Read the model definition and answer for the solid it produces. Units are mm, in the model's axes. A direction names the side the tool comes from. Coordinates: 2 decimals unless noted, no trailing zeros. Write each loop counter-clockwise with the first axis right and the second up, starting at its lowest first coordinate (ties: lowest second). Pieces come first, ordered by that corner, then holes. Notation, with made-up numbers: (88.5, -9.75) - (133.5, -9.75) arc R13 ccw to (133.5, 7.25) - close; hole circle Ø5 at (54, -21.75). An arc over 180 degrees is marked (long way). Use a Markdown table: item, result.
from build123d import *

# Parameters (mm, degrees)
F1_DEPTH = 171.45
F2_R     = 5.5626
F3_DEPTH = 72.873041
F4_R     = 3.9751
F5_DEPTH = 76.972204
F6_R     = 6.35


with BuildPart() as f1:
    # F0 (on Top) → F1 (new body)
    with BuildSketch(Plane.XY):
        with BuildLine():
            Line((0, 0), (0, 3.175))
            Line((0, 3.175), (-28.470279, 3.175))
            ThreePointArc((-28.470279, 3.175), (-30.537637, 3.520957), (-32.37973, 4.521132))
            Line((-32.37973, 4.521132), (-119.864904, 72.872041))
            Line((-119.864904, 72.872041), (-121.819629, 70.370107))
            Line((-121.819629, 70.370107), (-34.334455, 2.019198))
            ThreePointArc((-34.334455, 2.019198), (-31.571316, 0.518936), (-28.470279, 0))
            Line((-28.470279, 0), (0, 0))
        make_face()
    extrude(amount=F1_DEPTH)

    # F2 (on face) → F3 (cut, through all)
    with BuildSketch(Plane.XZ):
        with Locations((-15.875, 152.4)):
            Circle(F2_R)
        with Locations((-15.875, 38.1)):
            Circle(F2_R)
    extrude(amount=-F3_DEPTH, mode=Mode.SUBTRACT)

    # F4 (on face) → F5 (cut, through all)
    with BuildSketch(Plane(origin=(-12.03449, -15.403445, 0), x_dir=(0.788011, -0.615661, 0), z_dir=(-0.615661, -0.788011, 0))):
        with Locations((-128.194141, 81.28)):
            Circle(F4_R)
        with Locations((-42.469141, 81.28)):
            Circle(F4_R)
        with Locations((-42.469141, 25.4)):
            Circle(F4_R)
        with Locations((-128.194141, 25.4)):
            Circle(F4_R)
    extrude(amount=-F5_DEPTH, mode=Mode.SUBTRACT)

    # F6
    f6_edges = [f1.edges().sort_by_distance(p)[0] for p in [
        (-120.842267, 71.621074, 171.45),
        (-120.842267, 71.621074, 0),
        (0, 1.5875, 171.45),
        (0, 1.5875, 0),
    ]]
    fillet(f6_edges, radius=F6_R)


solid = f1.part
(1) A cutting plane is placed at D-D, the plane x = -101. Write down the section's boundary in (y, z), and give its area (3 significant figures).
Report:
| item | result |
|---|---|
| outline | (54.1, 0) - (58.13, 0) - (58.13, 171.45) - (54.1, 171.45) - close |
| area | 691 mm² |
(2) The mould has two halves that part along X. Classify faces 1 (the flat face through (-66, 30, 171.45)), 2 (the flat face through (-75.51, 38.22, 84.52)), 3 (the cylindrical face through (-17.08, 1.57, 146.97)): pulls with the +X half, pulls with the -X half, needs draft (parallel to the pull), parting line crosses it, or undercut.
Report:
| item | result |
|---|---|
| face 1 | needs draft |
| face 2 | pulls with the +X half |
| face 3 | undercut |
(3) Each of these flat-tipped pins is pushed along its axis until it touches: P1, Ø10, axis at x = -81, z = 93.5, coming from the +Y side; P2, Ø3, axis at y = 12.5, z = 111.5, coming from the -X side; P3, Ø2, axis at x = -62.5, z = 90.5, coming from the +Y side. Where does it stop, or does it pass through?
Report:
| item | result |
|---|---|
| P1 | stops at y = 46.41 |
| P2 | stops at x = -49.67 |
| P3 | stops at y = 28.83 |
(4) For faces 4 (the flat face through (-14, 3.175, 85)), 5 (the flat face through (-14, 0, 85)), determine the directions among +Z, -Z, +X, -X, +Y, -Y from which every point of the face is accessible in a straight line to the end or side of a thin tool.
Report:
| item | result |
|---|---|
| face 4 | +Z, -Z, +X, +Y |
| face 5 | +Z, -Z, +X, -X, -Y |
(5) A cutting plane is placed at B-B, the plane z = 57. Write down the section's boundary in (x, y) (3 decimals).
Report:
| item | result |
|---|---|
| outline | (-121.82, 70.37) - (-34.334, 2.019) arc R9.525 ccw to (-28.47, 0) - (0, 0) - (0, 3.175) - (-28.47, 3.175) arc R6.35 cw to (-32.38, 4.521) - (-119.865, 72.872) - close |
(6) A cutting plane is placed at A-A, the plane z = 38.1. Write down the section's boundary in (x, y) (3 decimals).
Report:
| item | result |
|---|---|
| outline | (-121.82, 70.37) - (-34.334, 2.019) arc R9.525 ccw to (-28.47, 0) - (-21.438, 0) - (-21.438, 3.175) - (-28.47, 3.175) arc R6.35 cw to (-32.38, 4.521) - (-119.865, 72.872) - close; (-10.312, 0) - (0, 0) - (0, 3.175) - (-10.312, 3.175) - close |
(7) A cutting plane is placed at C-C, the plane y = 38. Write down the section's boundary in (x, z), and give its area (3 significant figures).
Report:
| item | result |
|---|---|
| outline | (-80.39, 0) - (-75.23, 0) - (-75.23, 171.45) - (-80.39, 171.45) - close |
| area | 884 mm² |
(8) Straight lines are drawn through the part: L1, parallel to X at y = 32, z = 34; L2, parallel to Y at x = -46.5, z = 53; L3, parallel to X at y = 39, z = 130. For each, find the intervals that lie inside material, in ascending order.
Report:
| item | result |
|---|---|
| L1 | x = -72.71 to -67.55 |
| L2 | y = 11.52 to 15.55 |
| L3 | x = -81.67 to -76.51 |
